Print and shaded views of the part. All mm, measured from the part's lowest x, y and z. Coordinates: 2 decimals unless noted, no trailing zeros. Loops run counter-clockwise (first coordinate to the right, second up) from the corner with the lowest first, then second, coordinate; pieces in that order, holes last.
1) Saw through at C-C, the plane x = 50. Write the cut outline in (y, z) (3 decimals).
2) Pin check, flat tips, straight feed: pin 1 Ø1.6 at (y, z) = (62.5, 2.5) entering from -X; pin 2 Ø1 at (x, z) = (27, 1) entering from +Y. Stop position of each tip, or through.
3) Wall check: line 1 along X through (y, z) = (56.5, 1.1); line 2 along Y through (x, z) = (51, 2); line 3 along Y through (x, z) = (42, 2.2). Give the ranges that are in metal, low to high.
4) Saw through at A-A, the plane z = 1.8. Give the number of separate pieces and of enclosed holes in the cut face, and give its area (3 significant figures).
5) Saw through at B-B, the plane x = 76.2. Write the cut outline in (y, z) (3 decimals), and give its area (3 significant figures).
6) Saw through at D-D, the plane x = 12.5. Write the cut outline in (y, z) (3 decimals).
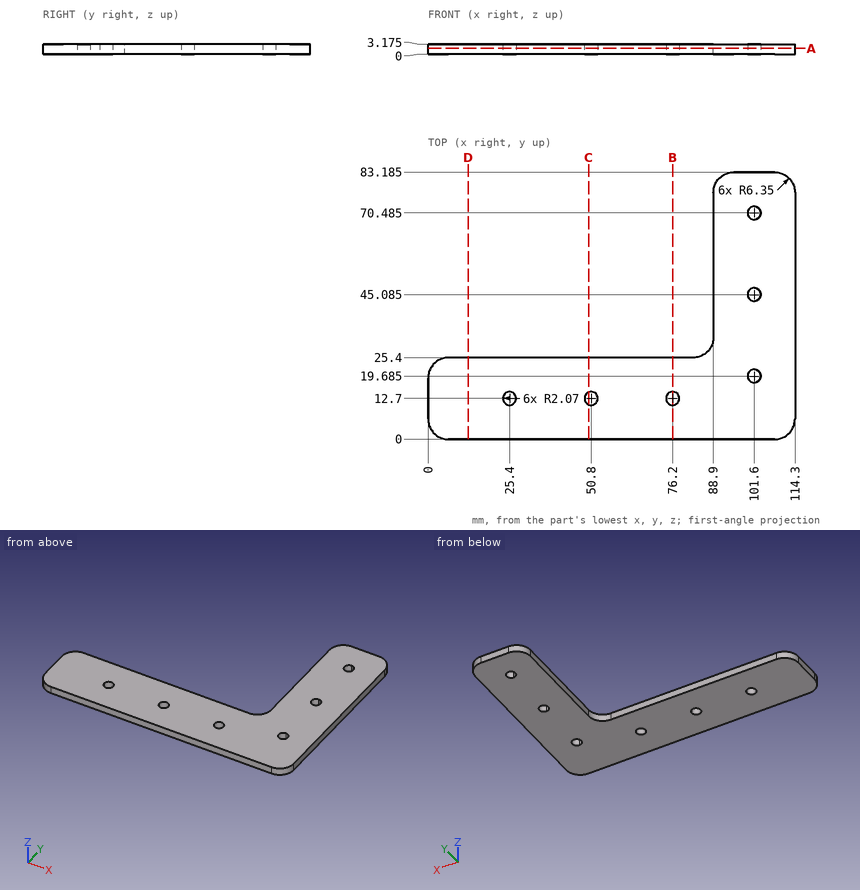
Data:
1. outline: (0, 0) - (10.791, 0) - (10.791, 3.175) - (0, 3.175) - close; (14.609, 0) - (25.4, 0) - (25.4, 3.175) - (14.609, 3.175) - close
2. pin 1: stops at x = 88.9
2. pin 2: stops at y = 25.4
3. line 1: x = 88.9 to 114.3
3. line 2: y = 0 to 10.64, 14.76 to 25.4
3. line 3: y = 0 to 25.4
4. separate pieces: 1
4. enclosed holes: 6
4. area: 4,260 mm2
5. outline: (0, 0) - (10.63, 0) - (10.63, 3.175) - (0, 3.175) - close; (14.77, 0) - (25.4, 0) - (25.4, 3.175) - (14.77, 3.175) - close
5. area: 67.5 mm2
6. outline: (0, 0) - (25.4, 0) - (25.4, 3.175) - (0, 3.175) - close
